Geometry check sheet. Reference: the model listing, model coordinates, mm. Give positions to 0.01 mm unless a question says otherwise; leave off trailing zeros. Loops run counter-clockwise (first coordinate to the right, second up) from the corner with the lowest first, then second, coordinate; pieces in that order, holes last. Notation, with made-up numbers: (54, 16.5) - (70, 16.5) arc R17 cw to (70, 37.5) - close; hole circle Ø8 at (74, 36). An arc over 180 degrees is marked (long way). Use a Markdown table: item, result. Add a question column.
1. Depth check by flat-ended pin: P1, Ø3, axis at x = -13.5, z = -553.5, coming from the +Y side; P2, Ø2, axis at y = -424.5, z = -473, coming from the -X side; P3, Ø11, axis at x = -14.5, y = -423.5, coming from the +Z side. Enter the tip coordinate at first touch or a pass-through.
2. Cross-section at A-A on y = -412. Enter the section's corners in (x, z), and give its area (3 significant figures).
3. Material ranges on L1, parallel to X at y = -442, z = -161.5, recorded low to high.
4. Cross-section at B-B on z = -859. Enter the section's corners in (x, y), and give its area (3 significant figures).
from build123d import *

# Parameters (mm, degrees)
SKETCH2_W           = 1000
SKETCH2_H           = 1000
BOSS_EXTRUDE2_DEPTH = 100
SKETCH4_W           = 145.74
SKETCH4_H           = 135.74
BOSS_EXTRUDE4_DEPTH = 8
FILLET1_R           = 10
SKETCH11_W          = 99.481944883
SKETCH11_H          = 99.481944883
BOSS_EXTRUDE6_DEPTH = 10
CUT_EXTRUDE2_DEPTH  = 199
FILLET5_R           = 5
SKETCH13_W          = 145.74
SKETCH13_H          = 10.277158346
CUT_EXTRUDE3_DEPTH  = 8
FILLET6_R           = 10


with BuildPart() as part:
    # Sketch2 → Boss-Extrude2 (new body)
    with BuildSketch(Plane(origin=(0, 0, 0), x_dir=(0, 0, -1), z_dir=(1, 0, 0))):
        with Locations((500, -500)):
            Rectangle(SKETCH2_W, SKETCH2_H)
    extrude(amount=BOSS_EXTRUDE2_DEPTH)

    # Sketch4 → Boss-Extrude4 (add)
    with BuildSketch(Plane.ZY):
        with Locations((-564.181498588, -429.969817094)):
            Rectangle(SKETCH4_W, SKETCH4_H)
    extrude(amount=BOSS_EXTRUDE4_DEPTH)

    # Fillet1
    fillet1_edges = [part.edges().sort_by_distance(p)[0] for p in [
        (-4, -362.099817094, -491.311498588),
        (-4, -362.099817094, -637.051498588),
        (-4, -497.839817094, -637.051498588),
        (-4, -497.839817094, -491.311498588),
    ]]
    fillet(fillet1_edges, radius=FILLET1_R)

    # Sketch11 → Boss-Extrude6 (add)
    with BuildSketch(Plane.ZY.offset(8)):
        with Locations((-562.051498588, -437.099817095)):
            Rectangle(SKETCH11_W, SKETCH11_H)
    extrude(amount=BOSS_EXTRUDE6_DEPTH)

    # Sketch12 → Cut-Extrude2 (cut)
    with BuildSketch(Plane(origin=(0, -486.840789536, 0), x_dir=(-1, 0, 0), z_dir=(0, -1, 0))):
        Polygon((8, 611.79247103), (18, 512.310526147), (18, 611.79247103), align=None)
    extrude(amount=-CUT_EXTRUDE2_DEPTH, mode=Mode.SUBTRACT)

    # Fillet5
    fillet5_edges = [part.edges().sort_by_distance(p)[0] for p in [
        (-13, -387.358844653, -512.310526147),
        (-13, -486.840789536, -512.310526147),
    ]]
    fillet(fillet5_edges, radius=FILLET5_R)

    # Sketch13 → Cut-Extrude3 (cut)
    with BuildSketch(Plane.ZY.offset(8)):
        with Locations((-564.181498588, -366.961237921)):
            Rectangle(SKETCH13_W, SKETCH13_H)
    extrude(amount=-CUT_EXTRUDE3_DEPTH, mode=Mode.SUBTRACT)

    # Fillet6
    fillet6_edges = [part.edges().sort_by_distance(p)[0] for p in [
        (-4, -372.099817094, -491.311498588),
        (-4, -372.099817094, -637.051498588),
    ]]
    fillet(fillet6_edges, radius=FILLET6_R)


solid = part.part
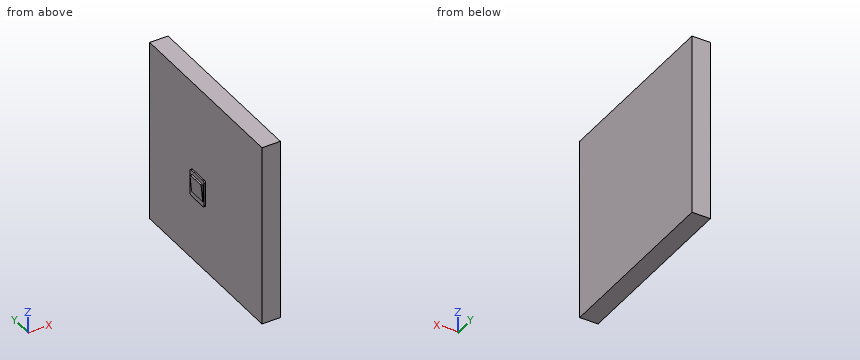
Values found:
| question | item | result |
|---|---|---|
| 1 | P1 | stops at y = -387.36 |
| 1 | P2 | stops at x = 0 |
| 1 | P3 | stops at z = -512.31 |
| 2 | outline | (-18, -512.31) - (-8, -611.79) - (-8, -637.05) - (0, -637.05) - (0, -1000) - (100, -1000) - (100, 0) - (0, 0) - (0, -491.31) - (-8, -491.31) - (-8, -512.31) - close |
| 2 | area | 102,000 mm2 |
| 3 | L1 | x = 0 to 100 |
| 4 | outline | (0, -1000) - (100, -1000) - (100, 0) - (0, 0) - close |
| 4 | area | 100,000 mm2 |
